```python
from build123d import *

# Parameters (mm, degrees)
BASE_FLANGE1_DEPTH      = 80
CUT_EXTRUDE1_DEPTH      = 219.463439317
CUT_EXTRUDE1_DEPTH_BACK = 219.463439317
SKETCH7_R               = 1.5
CUT_EXTRUDE3_DEPTH      = 0.7366
SKETCH8_R               = 1.5
CUT_EXTRUDE4_DEPTH      = 0.7366


# Sheet-metal steps are written as plain solids
with BuildPart() as part:
    # Sketch1 → Base-Flange1 (new body)
    with BuildSketch(Plane(origin=(0, 0, 0), x_dir=(1, 0, 0), z_dir=(0, 1, 0))):
        with BuildLine():
            Line((170, 55), (0.7, 55))
            ThreePointArc((0.7, 55), (0.205025253, 54.794974747), (0, 54.3))
            Line((0, 54.3), (0, 0))
            Line((0, 0), (0, -54.3))
            ThreePointArc((0, -54.3), (0.205025253, -54.794974747), (0.7, -55))
            Line((0.7, -55), (169, -55))
            Line((169, -55), (169, -55.7366))
            Line((169, -55.7366), (0.7, -55.7366))
            ThreePointArc((0.7, -55.7366), (-0.315829602, -55.315829602), (-0.7366, -54.3))
            Line((-0.7366, -54.3), (-0.7366, 0))
            Line((-0.7366, 0), (-0.7366, 54.3))
            ThreePointArc((-0.7366, 54.3), (-0.315829602, 55.315829602), (0.7, 55.7366))
            Line((0.7, 55.7366), (170, 55.7366))
            Line((170, 55.7366), (170, 55))
        make_face()
    extrude(amount=BASE_FLANGE1_DEPTH)

    # Sketch6 → Cut-Extrude1 (cut, two sides: drawn at the far end of the back side and taken through both)
    with BuildSketch(Plane.XY.offset(55.7366).offset(-CUT_EXTRUDE1_DEPTH_BACK)):
        Polygon((169, 50), (169, 0), (119, 0), align=None)
    extrude(amount=CUT_EXTRUDE1_DEPTH + CUT_EXTRUDE1_DEPTH_BACK, mode=Mode.SUBTRACT)

    # Sketch7 → Cut-Extrude3 (cut)
    with BuildSketch(Plane.XY.offset(55.7366)):
        with Locations((159, 70)):
            Circle(SKETCH7_R)
        with Locations((119, 70)):
            Circle(SKETCH7_R)
    extrude(amount=-CUT_EXTRUDE3_DEPTH, mode=Mode.SUBTRACT)

    # Sketch8 → Cut-Extrude4 (cut)
    with BuildSketch(Plane.XY.offset(-55.7366)):
        with Locations((140, 70)):
            Circle(SKETCH8_R)
    extrude(amount=CUT_EXTRUDE4_DEPTH, mode=Mode.SUBTRACT)


solid = part.part
```
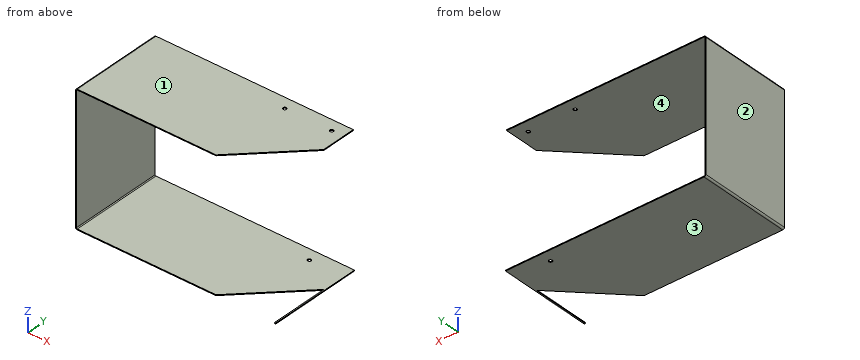
Could you check a few things on this model? Use its own coordinates, in mm. Face numbers are marked on the shaded views. Coordinates: 2 decimals unless noted, no trailing zeros. Write each loop counter-clockwise with the first axis right and the second up, starting at its lowest first coordinate (ties: lowest second). Pieces come first, ordered by that corner, then holes. Notation, with made-up numbers: (8, 43) -> (16, 43) arc R28 cw to (16, 75) -> close; hole circle Ø6 at (-3.5, 7). An arc over 180 degrees is marked (long way). Return JSON: item names as keys, results as strings.
(1) We'd pull the mould along Z, two halves only. Please class the marked faces 1, 2, 3 and 4: +Z half, -Z half, draft (parallel to the pull), parting line (faces both ways), or undercut.
Numbers:
{"face 1": "+Z half", "face 2": "draft", "face 3": "-Z half", "face 4": "undercut"}
(2) Imagine slicing it at A-A, the plane x = 29. Please give me the cut outline in (y, z).
Numbers:
{"outline": "(0, -55.74) -> (80, -55.74) -> (80, -55) -> (0, -55) -> close; (0, 55) -> (80, 55) -> (80, 55.74) -> (0, 55.74) -> close"}
(3) Imagine slicing it at B-B, the plane y = 20.5. Please give me the cut outline in (x, z).
Numbers:
{"outline": "(-0.74, -54.3) arc R1.44 ccw to (0.7, -55.74) -> (139.5, -55.74) -> (139.5, -55) -> (0.7, -55) arc R0.7 cw to (0, -54.3) -> (0, 54.3) arc R0.7 cw to (0.7, 55) -> (139.5, 55) -> (139.5, 55.74) -> (0.7, 55.74) arc R1.44 ccw to (-0.74, 54.3) -> close; (169, -55.74) -> (170, -55.74) -> (170, -55) -> (169, -55) -> close"}
(4) Imagine slicing it at C-C, the plane x = 126.5. Please give me the cut outline in (y, z).
Numbers:
{"outline": "(7.5, -55.74) -> (80, -55.74) -> (80, -55) -> (7.5, -55) -> close; (7.5, 55) -> (80, 55) -> (80, 55.74) -> (7.5, 55.74) -> close"}
(5) I need wall thicknesses on L1, parallel to X at y = 70, z = 55.35; L2, parallel to Z at x = 20, y = 59.5; L3, parallel to Y at x = 119, z = 55.1. Which ranges of each line are inside material? Lowest first, please.
Numbers:
{"L1": "x = -0.28 to 117.5, 120.5 to 157.5, 160.5 to 169", "L2": "z = -55.74 to -55, 55 to 55.74", "L3": "y = 0 to 68.5, 71.5 to 80"}
(6) Imagine slicing it at D-D, the plane y = 40. Please give me the cut outline in (x, z).
Numbers:
{"outline": "(-0.74, -54.3) arc R1.44 ccw to (0.7, -55.74) -> (159, -55.74) -> (159, -55) -> (0.7, -55) arc R0.7 cw to (0, -54.3) -> (0, 54.3) arc R0.7 cw to (0.7, 55) -> (159, 55) -> (159, 55.74) -> (0.7, 55.74) arc R1.44 ccw to (-0.74, 54.3) -> close; (169, -55.74) -> (170, -55.74) -> (170, -55) -> (169, -55) -> close"}
(7) I'm going to push flat-ended pins straight in: pin 1 (4 mm diameter, centred on x = 119, y = 70, fed in from +Z); pin 2 (1.8 mm diameter, centred on x = 159, y = 70, fed in from +Z). Where does each tip first touch, or does it pass through?
Numbers:
{"pin 1": "stops at z = 55.74", "pin 2": "stops at z = -55"}
